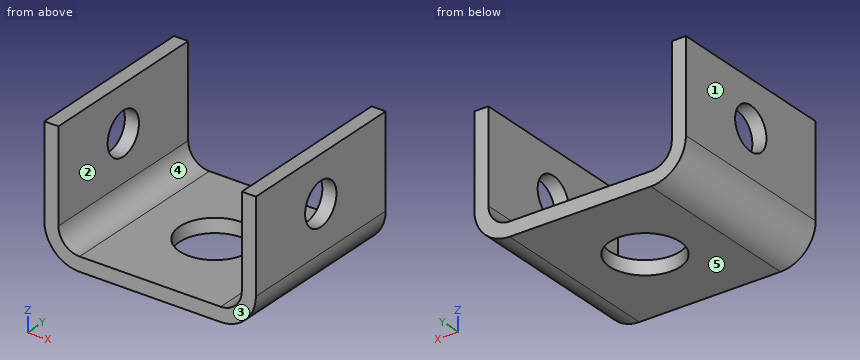
from build123d import *

# Parameters (mm, degrees)
BASE_FLANGE2_DEPTH      = 12.5
CUT_EXTRUDE2_DEPTH      = 38.151715977
CUT_EXTRUDE2_DEPTH_BACK = 38.151715977
SKETCH11_R              = 3.018390671
CUT_EXTRUDE3_REACH      = 28.557
SKETCH13_R              = 5


# Sheet-metal steps are written as plain solids
with BuildPart() as part:
    # Sketch2 → Base-Flange2 (new, symmetric)
    with BuildSketch(Plane(origin=(0, 0, 0), x_dir=(1, 0, 0), z_dir=(0, 1, 0))):
        with BuildLine():
            Line((-15, 0), (-15, 13))
            ThreePointArc((-15, 13), (-13.535533906, 16.535533906), (-10, 18))
            Line((-10, 18), (10, 18))
            ThreePointArc((10, 18), (13.535533906, 16.535533906), (15, 13))
            Line((15, 13), (15, 0))
            Line((15, 0), (13, 0))
            Line((13, 0), (13, 13))
            ThreePointArc((13, 13), (12.121320344, 15.121320344), (10, 16))
            Line((10, 16), (-10, 16))
            ThreePointArc((-10, 16), (-12.121320344, 15.121320344), (-13, 13))
            Line((-13, 13), (-13, 0))
            Line((-13, 0), (-15, 0))
        make_face()
    extrude(amount=BASE_FLANGE2_DEPTH, both=True)

    # Sketch11 → Cut-Extrude2 (cut, two sides: drawn at the far end of the back side and taken through both)
    with BuildSketch(Plane(origin=(15, 0, 0), x_dir=(0, 0, -1), z_dir=(1, 0, 0)).offset(-CUT_EXTRUDE2_DEPTH_BACK)):
        with Locations(Location((6.5, 0, 0), (0, 0, 180))):
            Circle(SKETCH11_R)
    extrude(amount=CUT_EXTRUDE2_DEPTH + CUT_EXTRUDE2_DEPTH_BACK, mode=Mode.SUBTRACT)

    # Sketch13 → Cut-Extrude3 (cut, up to next)
    with BuildSketch(Plane(origin=(0, 0, -18), x_dir=(-1, 0, 0), z_dir=(0, 0, -1)), mode=Mode.PRIVATE) as cut_extrude3_sk1:
        Circle(SKETCH13_R)
    cut_extrude3_tool1 = extrude(cut_extrude3_sk1.sketch, amount=-CUT_EXTRUDE3_REACH, mode=Mode.PRIVATE) & part.part
    add(cut_extrude3_tool1.solids().sort_by_distance((0, 0, -18))[0], mode=Mode.SUBTRACT)


solid = part.part
Model file for the job. Use its own axes, mm. Face numbers are marked on the shaded views. A direction names the side the tool comes from. Give positions to 0.01 mm unless a question says otherwise; leave off trailing zeros. Loops run counter-clockwise (first coordinate to the right, second up) from the corner with the lowest first, then second, coordinate; pieces in that order, holes last. Notation, with made-up numbers: (8.5, 46) -> (49.5, 46) arc R29 ccw to (49.5, 79) -> close; hole circle Ø10 at (67.5, 79.25). An arc over 180 degrees is marked (long way). Use a Markdown table: item, result. Add a question column.
(1) Slice it at A-A on z = -6.5. List the corners of the cut face in (x, y), and give its area (3 significant figures).
(2) Drop a flat-ended pin along its axis: pin 1 Ø6 at (x, y) = (9, -8) entering from +Z. Give the stop position or say it passes through.
(3) Slice it at C-C on x = 0. List the corners of the cut face in (y, z), and give its area (3 significant figures).
(4) Slice it at B-B on y = 0. List the corners of the cut face in (x, z), and give its area (3 significant figures).
(5) Wall check: line 1 along X through (y, z) = (2.75, -10.25); line 2 along Y through (x, z) = (-14.2, -6.5); line 3 along Y through (x, z) = (0, -17.6). Give the ranges that are in metal, low to high.
(6) Mould opens along X. For the marked faces 1, 2 and 3 say: +X half, -X half, draft (parallel to the pull), parting line (faces both ways), or undercut.
(7) Tool access for the marked faces 4 and 5: list every direction of +Z, -Z, +X, -X, +Y, -Y with a clear straight run to the whole face (end or side of a thin tool).
(8) Slice it at D-D on z = -1. List the corners of the cut face in (x, y), and give its area (3 significant figures).
Filled sheet:
| question | item | result |
|---|---|---|
| 1 | outline | (-15, -12.5) -> (-13, -12.5) -> (-13, -3.02) -> (-15, -3.02) -> close; (-15, 3.02) -> (-13, 3.02) -> (-13, 12.5) -> (-15, 12.5) -> close; (13, -12.5) -> (15, -12.5) -> (15, -3.02) -> (13, -3.02) -> close; (13, 3.02) -> (15, 3.02) -> (15, 12.5) -> (13, 12.5) -> close |
| 1 | area | 75.9 mm2 |
| 2 | pin 1 | z = -15.24 |
| 3 | outline | (-12.5, -18) -> (-5, -18) -> (-5, -16) -> (-12.5, -16) -> close; (5, -18) -> (12.5, -18) -> (12.5, -16) -> (5, -16) -> close |
| 3 | area | 30.0 mm2 |
| 4 | outline | (-15, -13) arc R5 ccw to (-10, -18) -> (-5, -18) -> (-5, -16) -> (-10, -16) arc R3 cw to (-13, -13) -> (-13, -9.52) -> (-15, -9.52) -> close; (-15, -3.48) -> (-13, -3.48) -> (-13, 0) -> (-15, 0) -> close; (5, -18) -> (10, -18) arc R5 ccw to (15, -13) -> (15, -9.52) -> (13, -9.52) -> (13, -13) arc R3 cw to (10, -16) -> (5, -16) -> close; (13, -3.48) -> (15, -3.48) -> (15, 0) -> (13, 0) -> close |
| 4 | area | 73.0 mm2 |
| 5 | line 1 | -15 to -13, 13 to 15 |
| 5 | line 2 | -12.5 to -3.02, 3.02 to 12.5 |
| 5 | line 3 | -12.5 to -5, 5 to 12.5 |
| 6 | face 1 | -X half |
| 6 | face 2 | undercut |
| 6 | face 3 | draft |
| 7 | face 4 | +Z, +Y, -Y |
| 7 | face 5 | -Z, +X, -X, +Y, -Y |
| 8 | outline | (-15, -12.5) -> (-13, -12.5) -> (-13, 12.5) -> (-15, 12.5) -> close; (13, -12.5) -> (15, -12.5) -> (15, 12.5) -> (13, 12.5) -> close |
| 8 | area | 100 mm2 |
